```python
from build123d import *

# Parameters (mm, degrees)
F0_W     = 25
F0_H     = 25
F1_DEPTH = 40
F2_R     = 10.5
F3_DEPTH = 30
F4_R     = 2.25
F5_DEPTH = 25
F6_W     = 3
F6_H     = 7
F7_DEPTH = 25
F8_R     = 9.526155
F9_DEPTH = 9


with BuildPart() as f1:
    # F0 (on Top) → F1 (new body)
    with BuildSketch(Plane.XY):
        Rectangle(F0_W, F0_H)
    extrude(amount=F1_DEPTH)

    # F2 (on face) → F3 (cut)
    with BuildSketch(Plane.XY.offset(40)):
        Circle(F2_R)
    extrude(amount=-F3_DEPTH, mode=Mode.SUBTRACT)

    # F4 (on face) → F5 (cut)
    with BuildSketch(Plane.XY.offset(10)):
        Circle(F4_R)
    extrude(amount=-F5_DEPTH, mode=Mode.SUBTRACT)

    # F6 (on face) → F7 (cut)
    with BuildSketch(Plane.YZ.offset(12.5)):
        with Locations((0, 36.5)):
            Rectangle(F6_W, F6_H)
    extrude(amount=-F7_DEPTH, mode=Mode.SUBTRACT)

    # F8 (on face) → F9 (cut)
    with BuildSketch(Plane.XY.offset(10)):
        with Locations((0, -0.073845)):
            Circle(F8_R)
    extrude(amount=-F9_DEPTH, mode=Mode.SUBTRACT)


solid = f1.part
```
Source: CAD feature listing. Evaluate the final solid. Frame: model axes, mm. A direction names the side the tool comes from. Give positions to 0.01 mm unless a question says otherwise; leave off trailing zeros. Loops run counter-clockwise (first coordinate to the right, second up) from the corner with the lowest first, then second, coordinate; pieces in that order, holes last. Notation, with made-up numbers: (19, 20) -> (73, 20) arc R35 cw to (73, 52) -> close; hole circle Ø10 at (-25, 60). An arc over 180 degrees is marked (long way). Put each result on its own line as item: value. Start each with the question number.
1) Draft query along X for faces 1 (the face through (12.5, 0, 20)), 2 (the face through (11, 1.5, 36)), 3 (the face through (-0.29, 2.23, 0.51)). Return one class per face: released by +X, released by -X, zero draft, split by the parting line, or undercut.
2) Cut plane B-B (x = 0). Return loops of the section in (y, z), then the cut area to 3 significant figures.
3) Contact query for flat-ended pins moving along their axis: P1, Ø15, axis at x = 0, y = -0.07, coming from the +Z side; P2, Ø1.7, axis at x = 11, y = -0.5, coming from the +Z side; P3, Ø2.5, axis at x = 0, y = 0, coming from the +Z side. Output: stop coordinate, or through.
4) Material intervals for probe 1 along Y at (x, z) = (0, 4.25); probe 2 along Y at (x, z) = (0, 23.5); probe 3 along X at (y, z) = (-1.5, 17), sorted ascending.
5) Cut plane A-A (z = 36). Return loops of the section in (x, y).
6) Cut plane D-D (x = 5.5). Return loops of the section in (y, z), then the cut area to 3 significant figures.
7) Reachability of faces 4 (the face through (11, 0, 33)), 5 (the face through (-4, 9, 10)), 6 (the face through (0, 12.5, 20)) from +Z, -Z, +X, -X, +Y, -Y: full face, straight path, thin tool, end or side. Return the list, or none.
8) Cut plane C-C (z = 16). Return loops of the section in (x, y).
Results are:
1. face 1: released by +X
1. face 2: zero draft
1. face 3: undercut
2. outline: (-12.5, 0) -> (-2.25, 0) -> (-2.25, 1) -> (-9.6, 1) -> (-9.6, 10) -> (-10.5, 10) -> (-10.5, 40) -> (-12.5, 40) -> close; (2.25, 0) -> (12.5, 0) -> (12.5, 40) -> (10.5, 40) -> (10.5, 10) -> (9.45, 10) -> (9.45, 1) -> (2.25, 1) -> close
2. area: 194 mm2
3. P1: stops at z = 1
3. P2: stops at z = 33
3. P3: passes through
4. probe 1: y = -12.5 to -9.6, 9.45 to 12.5
4. probe 2: y = -12.5 to -10.5, 10.5 to 12.5
4. probe 3: x = -12.5 to -10.39, 10.39 to 12.5
5. outline: (-12.5, -12.5) -> (12.5, -12.5) -> (12.5, -1.5) -> (10.39, -1.5) arc R10.5 cw to (-10.39, -1.5) -> (-12.5, -1.5) -> close; (-12.5, 1.5) -> (-10.39, 1.5) arc R10.5 cw to (10.39, 1.5) -> (12.5, 1.5) -> (12.5, 12.5) -> (-12.5, 12.5) -> close
6. outline: (-12.5, 0) -> (12.5, 0) -> (12.5, 40) -> (8.94, 40) -> (8.94, 10) -> (7.7, 10) -> (7.7, 1) -> (-7.85, 1) -> (-7.85, 10) -> (-8.94, 10) -> (-8.94, 40) -> (-12.5, 40) -> close
6. area: 323 mm2
7. face 4: +Z, +X, -X
7. face 5: +Z
7. face 6: +Z, -Z, +X, -X, +Y
8. outline: (-12.5, -12.5) -> (12.5, -12.5) -> (12.5, 12.5) -> (-12.5, 12.5) -> close; hole circle Ø21 at (0, 0)
